Source: CAD feature listing. Evaluate the final solid. Frame: model axes, mm. Coordinates: 2 decimals unless noted, no trailing zeros. Order: outer loops, then holes, each group sorted by start corner. A loop starts at its lowest first (then second) coordinate and runs counter-clockwise, first axis right, second up.
```python
from build123d import *

# Parameters (mm, degrees)
SKETCH1_R           = 4.25
BOSS_EXTRUDE1_DEPTH = 60
SKETCH2_R           = 0.5
BOSS_EXTRUDE2_DEPTH = 0.1
CIRPATTERN1_COUNT   = 4


with BuildPart() as part:
    # Sketch1 → Boss-Extrude1 (new body)
    with BuildSketch(Plane.XY):
        with Locations(Location((0, 0, 0), (0, 0, 180))):
            Circle(SKETCH1_R)
    extrude(amount=BOSS_EXTRUDE1_DEPTH)

    # Sketch2 → Boss-Extrude2 (add)
    with BuildSketch(Plane(origin=(0, 0, 0), x_dir=(-1, 0, 0), z_dir=(0, 0, -1))):
        with Locations(Location((-1, 3, 0), (0, 0, 180))):
            Circle(SKETCH2_R)
        with Locations(Location((1, 3, 0), (0, 0, 180))):
            Circle(SKETCH2_R)
    boss_extrude2 = extrude(amount=BOSS_EXTRUDE2_DEPTH)

    # CirPattern1: Boss-Extrude2 ×4 about axis
    cirpattern1_axis = Axis((0, 0, 0), (0, 0, 1))
    for i in range(1, CIRPATTERN1_COUNT):
        add(boss_extrude2.rotate(cirpattern1_axis, i * 360 / CIRPATTERN1_COUNT))


solid = part.part
```
1. Pin query (flat end, axial travel): P1, Ø2, axis at x = -0.5, y = -1, coming from the -Z side; P2, Ø4, axis at x = 3, y = -3.5, coming from the -Z side; P3, Ø2, axis at x = -3, z = 26, coming from the -Y side; P4, Ø3, axis at x = -2.5, z = 8, coming from the -Y side. Return the tip coordinate at first contact, or that it passes through.
Findings:
P1: stops at z = 0
P2: stops at z = -0.1
P3: stops at y = -3.75
P4: stops at y = -4.13
2. Draft query along X for faces 1 (the face through (1, 3, -0.1)), 2 (the face through (0, 0, 0)), 3 (the face through (0.553, -4.214, 29.58)). Return one class per face: released by +X, released by -X, zero draft, split by the parting line, or undercut.
Findings:
face 1: zero draft
face 2: undercut
face 3: split by the parting line
3. Section query D-D on x = -1. Return loops of the section in (y, z), plus the area to 3 significant figures.
Findings:
outline: (-4.13, 0) - (-3.5, 0) - (-3.5, -0.1) - (-2.5, -0.1) - (-2.5, 0) - (2.5, 0) - (2.5, -0.1) - (3.5, -0.1) - (3.5, 0) - (4.13, 0) - (4.13, 60) - (-4.13, 60) - close
area: 496 mm2
4. Section query C-C on z = 13. Return loops of the section in (x, y), plus the area to 3 significant figures.
Findings:
outline: circle Ø8.5 at (0, 0)
area: 56.7 mm2
5. Section query B-B on x = 3. Return loops of the section in (y, z), plus the area to 3 significant figures.
Findings:
outline: (-3.01, 0) - (-1.5, 0) - (-1.5, -0.1) - (-0.5, -0.1) - (-0.5, 0) - (0.5, 0) - (0.5, -0.1) - (1.5, -0.1) - (1.5, 0) - (3.01, 0) - (3.01, 60) - (-3.01, 60) - close
area: 361 mm2
6. Section query A-A on y = -2. Return loops of the section in (x, z), plus the area to 3 significant figures.
Findings:
outline: (-3.75, 0) - (3.75, 0) - (3.75, 60) - (-3.75, 60) - close
area: 450 mm2
7. Ray query, line 1 (Z direction, x = 3.5, y = 1.25); line 2 (X direction, y = -0.25, z = 25.5); line 3 (X direction, y = -2, z = 10.5). Return the intervals inside material, ascending.
Findings:
line 1: z = 0 to 60
line 2: x = -4.24 to 4.24
line 3: x = -3.75 to 3.75
